Part print with two shaded views. Sizes in mm from the minimum x, y, z corner. Round coordinates to 2 decimals unless told otherwise and drop trailing zeros. Write each loop counter-clockwise with the first axis right and the second up, starting at its lowest first coordinate (ties: lowest second). Pieces come first, ordered by that corner, then holes. Notation, with made-up numbers: (64, 49.5) - (104, 49.5) arc R32 cw to (104, 81.5) - close; hole circle Ø9 at (53, -18). An arc over 180 degrees is marked (long way). Use one line per item in the form item = value. Start each with the question number.
Item 1: Drill centre lines: L1, parallel to X at y = 0.65, z = 24; L2, parallel to Z at x = 24, y = 1.1; L3, parallel to X at y = 1, z = 35.5. Where is each one in solid material? Low to high.
Item 2: Band-saw the part on D-D, the plane z = 40. List the corners of the cut face in (x, y), and give its area (3 significant figures).
Item 3: Band-saw the part on C-C, the plane y = 0.5. List the corners of the cut face in (x, z).
Item 4: Band-saw the part on B-B, the plane z = 24. List the corners of the cut face in (x, y).
Item 5: Band-saw the part on A-A, the plane x = 24. List the corners of the cut face in (y, z).
Item 6: Pin check, flat tips, straight feed: pin 1 (6 mm diameter, centred on x = 32, z = 15.5, fed in from +Y); pin 2 (0.6 mm diameter, centred on x = 5.5, y = 1, fed in from +Z); pin 3 (3 mm diameter, centred on x = 32.5, z = 35.5, fed in from +Y); pin 4 (0.6 mm diameter, centred on y = 0.5, z = 41.5, fed in from -X). Stop position of each tip, or through.
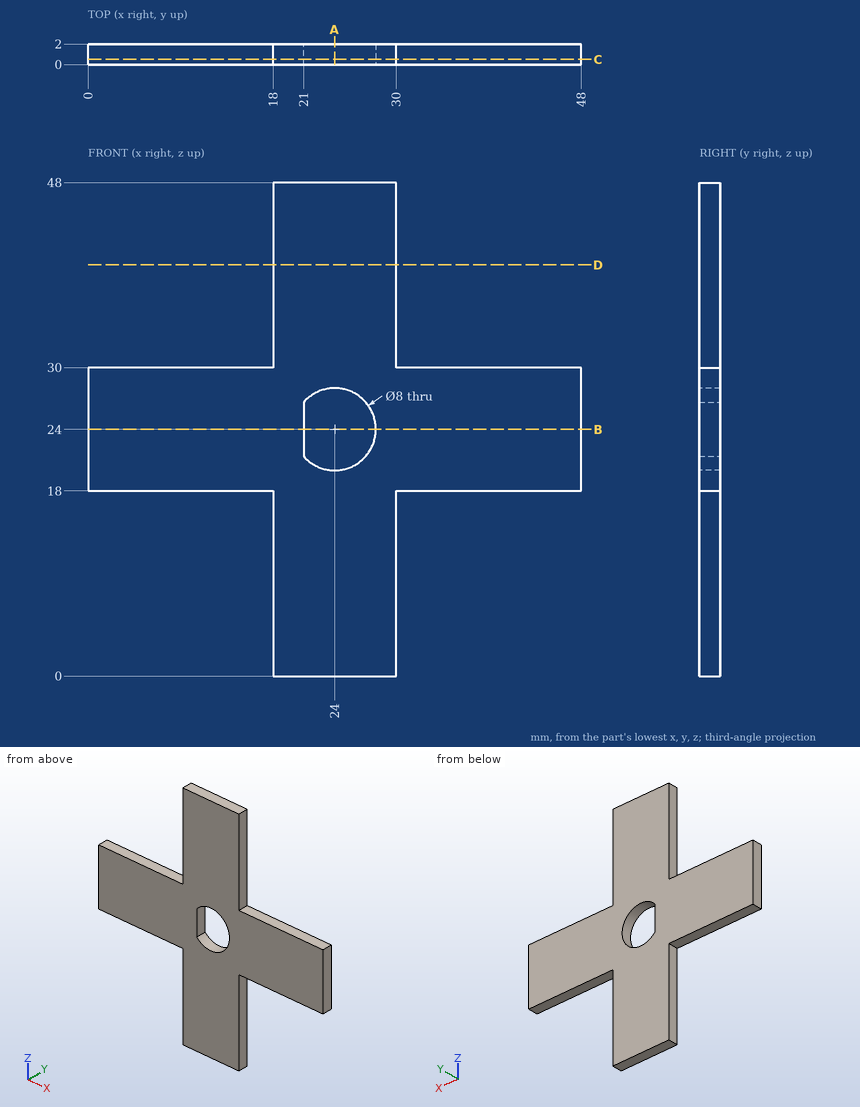
Determined:
q1.L1 = 0 to 21, 28 to 48
q1.L2 = 0 to 20, 28 to 48
q1.L3 = 18 to 30
q2.outline = (18, 0) - (30, 0) - (30, 2) - (18, 2) - close
q2.area = 24.0 mm²
q3.outline = (0, 18) - (18, 18) - (18, 0) - (30, 0) - (30, 18) - (48, 18) - (48, 30) - (30, 30) - (30, 48) - (18, 48) - (18, 30) - (0, 30) - close; hole (21, 21.35) arc R4 ccw (long way) to (21, 26.65) - close
q4.outline = (0, 0) - (21, 0) - (21, 2) - (0, 2) - close; (28, 0) - (48, 0) - (48, 2) - (28, 2) - close
q5.outline = (0, 0) - (2, 0) - (2, 20) - (0, 20) - close; (0, 28) - (2, 28) - (2, 48) - (0, 48) - close
q6.pin_1 = 2
q6.pin_2 = 30
q6.pin_3 = through
q6.pin_4 = 18
